Input: part model. Units: mm. Frame: model coordinates. Round coordinates to 2 decimals unless told otherwise and drop trailing zeros. Loops run counter-clockwise (first coordinate to the right, second up) from the corner with the lowest first, then second, coordinate; pieces in that order, holes last. Notation, with made-up numbers: M -15,37 L 37,37 A12 cw 37,49 Z; hole C -15.75,41 d10. An arc over 180 degrees is marked long. Use one line per item in the form item = value. Start each with the question number.
Q1. Mould query, pull axis X, two halves, no side actions, for faces 1 (the cylindrical face through (495, -10, 0)), 2 (the cylindrical face through (465.58, 7.81, -1.73)). Classes: pulls with the +X half, pulls with the -X half, needs draft (parallel to the pull), parting line crosses it, or undercut.
Q2. Ray query, line 1 along Y through (x, z) = (-100, 0); line 2 along X through (y, z) = (-4.5, -11); line 3 along Y through (x, z) = (-96, 0). Return the intervals inside material, ascending.
Q3. Section query A-A, the plane x = 244. Output: boundary loops of the cut face in (y, z), and give its area (3 significant figures).
Q4. First-contact query: P1, Ø6.5, axis at y = 4.64, z = -14.27, coming from the +X side; P2, Ø2, axis at x = 383, z = -3, coming from the +Y side; P3, Ø2, axis at x = -16.5, z = 10, coming from the +Y side. Flat tips, straight axial feed; report the tip coordinate or a pass-through.
```python
from build123d import *

# Parameters (mm, degrees)
SKETCH1_R             = 8
BOSS_EXTRUDE1_DEPTH   = 47.5
BOSS_EXTRUDE2_START   = 15
BOSS_EXTRUDE2_DEPTH   = 10
SKETCH3_R             = 9
BOSS_EXTRUDE3_DEPTH   = 4
LPATTERN1_COUNT       = 6
LPATTERN1_PITCH       = 95
BODY_MOVE_COPY1_ANGLE = 60
BODY_MOVE_COPY3_ANGLE = 120
BODY_MOVE_COPY4_ANGLE = 60
BODY_MOVE_COPY5_ANGLE = 120
BODY_MOVE_COPY6_ANGLE = 180
BOSS_EXTRUDE4_START   = 5
SKETCH4_R             = 9
BOSS_EXTRUDE4_DEPTH   = 5
SKETCH5_R             = 7.5
BOSS_EXTRUDE5_DEPTH   = 5
SKETCH6_R             = 8
BOSS_EXTRUDE6_DEPTH   = 7.5
SKETCH7_R             = 9
BOSS_EXTRUDE7_DEPTH   = 5
SKETCH8_R             = 8
BOSS_EXTRUDE8_DEPTH   = 38
SKETCH10_R            = 25
SKETCH10_R_2          = 2.5
BOSS_EXTRUDE9_DEPTH   = 10
SKETCH11_R            = 2.5
CUT_EXTRUDE1_DEPTH    = 15
FILLET1_R             = 2


with BuildPart() as part:
    # Sketch1 → Boss-Extrude1 (new, symmetric)
    with BuildSketch(Plane(origin=(0, 0, 0), x_dir=(0, 0, -1), z_dir=(1, 0, 0))):
        Circle(SKETCH1_R)
    extrude(amount=BOSS_EXTRUDE1_DEPTH, both=True)

    # Sketch2 → Boss-Extrude2 (add)
    with BuildSketch(Plane(origin=(0, 0, 0), x_dir=(0, 0, -1), z_dir=(1, 0, 0)).offset(BOSS_EXTRUDE2_START)):
        with BuildLine():
            Line((-8.746197071, -4.848096202), (-5.540743078, -12.343398625))
            ThreePointArc((-5.540743078, -12.343398625), (0, -16), (5.540743078, -12.343398625))
            Line((5.540743078, -12.343398625), (8.746197071, -4.848096202))
            ThreePointArc((8.746197071, -4.848096202), (0, 10), (-8.746197071, -4.848096202))
        make_face()
    boss_extrude2 = extrude(amount=BOSS_EXTRUDE2_DEPTH)

    # Mirror1: Boss-Extrude2 across plane
    add(boss_extrude2.mirror(Plane(origin=(0, 0, 0), x_dir=(0, 0, 1), z_dir=(1, 0, 0))))

    # Sketch3 → Boss-Extrude3 (add, symmetric)
    with BuildSketch(Plane(origin=(0, 0, 0), x_dir=(0, 0, -1), z_dir=(1, 0, 0))):
        Circle(SKETCH3_R)
    extrude(amount=BOSS_EXTRUDE3_DEPTH, both=True)


with BuildPart() as lpattern1_1:
    # LPattern1: pattern copy
    add(part.part.moved(Location(Vector(1, 0, 0) * (1 * LPATTERN1_PITCH))))


with BuildPart() as lpattern1_2:
    # LPattern1: pattern copy
    add(part.part.moved(Location(Vector(1, 0, 0) * (2 * LPATTERN1_PITCH))))


with BuildPart() as lpattern1_3:
    # LPattern1: pattern copy
    add(part.part.moved(Location(Vector(1, 0, 0) * (3 * LPATTERN1_PITCH))))


with BuildPart() as lpattern1_4:
    # LPattern1: pattern copy
    add(part.part.moved(Location(Vector(1, 0, 0) * (4 * LPATTERN1_PITCH))))


with BuildPart() as lpattern1_5:
    # LPattern1: pattern copy
    add(part.part.moved(Location(Vector(1, 0, 0) * (5 * LPATTERN1_PITCH))))


with BuildPart() as lpattern1_3_1:
    # Body-Move/Copy1: moved
    add(lpattern1_3.part.rotate(Axis((0, 0, 0), (-1, 0, 0)), BODY_MOVE_COPY1_ANGLE))


with BuildPart() as lpattern1_1_1:
    # Body-Move/Copy3: moved
    add(lpattern1_1.part.rotate(Axis((0, 0, 0), (-1, 0, 0)), BODY_MOVE_COPY3_ANGLE))


with BuildPart() as lpattern1_4_1:
    # Body-Move/Copy4: moved
    add(lpattern1_4.part.rotate(Axis((0, 0, 0), (1, 0, 0)), BODY_MOVE_COPY4_ANGLE))


with BuildPart() as lpattern1_2_1:
    # Body-Move/Copy5: moved
    add(lpattern1_2.part.rotate(Axis((0, 0, 0), (1, 0, 0)), BODY_MOVE_COPY5_ANGLE))


with BuildPart() as lpattern1_5_1:
    # Body-Move/Copy6: moved
    add(lpattern1_5.part.rotate(Axis((0, 0, 0), (1, 0, 0)), BODY_MOVE_COPY6_ANGLE))

    # Sketch4 → Boss-Extrude4 (add)
    with BuildSketch(Plane(origin=(522.5, 0, 0), x_dir=(0, 0, -1), z_dir=(1, 0, 0)).offset(BOSS_EXTRUDE4_START)):
        Circle(SKETCH4_R)
    extrude(amount=-BOSS_EXTRUDE4_DEPTH)

    # Combine1: union LPattern1_3, LPattern1_4, LPattern1_2, LPattern1_1, part
    add(lpattern1_3_1.part)
    add(lpattern1_4_1.part)
    add(lpattern1_2_1.part)
    add(lpattern1_1_1.part)
    add(part.part)

    # Sketch5 → Boss-Extrude5 (add)
    with BuildSketch(Plane(origin=(527.5, 0, 0), x_dir=(0, 0, -1), z_dir=(1, 0, 0))):
        Circle(SKETCH5_R)
    extrude(amount=BOSS_EXTRUDE5_DEPTH)

    # Sketch6 → Boss-Extrude6 (add)
    with BuildSketch(Plane.ZY.offset(47.5)):
        Circle(SKETCH6_R)
    extrude(amount=BOSS_EXTRUDE6_DEPTH)

    # Sketch7 → Boss-Extrude7 (add)
    with BuildSketch(Plane.ZY.offset(55)):
        Circle(SKETCH7_R)
    extrude(amount=BOSS_EXTRUDE7_DEPTH)

    # Sketch8 → Boss-Extrude8 (add)
    with BuildSketch(Plane.ZY.offset(60)):
        Circle(SKETCH8_R)
    extrude(amount=BOSS_EXTRUDE8_DEPTH)

    # Sketch10 → Boss-Extrude9 (add)
    with BuildSketch(Plane.ZY.offset(98)):
        Circle(SKETCH10_R)
        Circle(SKETCH10_R_2, mode=Mode.SUBTRACT)
    extrude(amount=BOSS_EXTRUDE9_DEPTH)

    # Sketch11 → Cut-Extrude1 (cut)
    with BuildSketch(Plane.ZY.offset(108)):
        Circle(SKETCH11_R)
        with Locations((0, 15)):
            Circle(SKETCH11_R)
        with Locations((14.265847744, 4.635254916)):
            Circle(SKETCH11_R)
        with Locations((8.816778784, -12.135254916)):
            Circle(SKETCH11_R)
        with Locations((-8.816778784, -12.135254916)):
            Circle(SKETCH11_R)
        with Locations((-14.265847744, 4.635254916)):
            Circle(SKETCH11_R)
    extrude(amount=-CUT_EXTRUDE1_DEPTH, mode=Mode.SUBTRACT)

    # Fillet1
    fillet1_edges = [lpattern1_5_1.edges().sort_by_distance(p)[0] for p in [
        (-98, 0, -8),
        (-98, 0, -25),
    ]]
    fillet(fillet1_edges, radius=FILLET1_R)


solid = lpattern1_5_1.part
```
Results found:
q1.face_1 = needs draft
q1.face_2 = undercut
q2.line_1 = -25 to -2.5, 2.5 to 12.5, 17.5 to 25
q2.line_2 = -108 to -98, 355 to 365, 395 to 405
q2.line_3 = -8 to -2.5, 2.5 to 8
q3.outline = C 0,0 d16
q3.area = 201 mm²
q4.P1 = 215
q4.P2 = 8.77
q4.P3 = 4.36
